Part model, mm, in its own coordinate system. A direction names the side the tool comes from. Coordinates: 2 decimals unless noted, no trailing zeros. Write each loop counter-clockwise with the first axis right and the second up, starting at its lowest first coordinate (ties: lowest second). Pieces come first, ordered by that corner, then holes. Notation, with made-up numbers: (63.25, -14.5) - (86.25, -14.5) arc R3 ccw to (86.25, -10.5) - close; hole circle Ø11 at (76.5, -39.5). An arc over 180 degrees is marked (long way). Write each question's results on one line, items separated by ' | '.
from build123d import *

# Parameters (mm, degrees)
F1_DEPTH = 88.9
F2_W     = 6.731
F2_H     = 6.731
F3_DEPTH = 49.5578889657
F4_ANGLE = 45
F5_ANGLE = 90
F6_ANGLE = 90


with BuildPart() as f1:
    # F0 (on Top) → F1 (new body)
    with BuildSketch(Plane.XY):
        Polygon((-10.7315, -10.7315), (-10.7315, 10.2235), (10.2235, 10.2235), (17.0815, 17.0815), (-0.8790122421, 35.0420122421), (-35.0420122421, 0.8790122421), (-17.0815, -17.0815), align=None)
    extrude(amount=F1_DEPTH)

    # F2 (on face) → F3 (cut, through all)
    with BuildSketch(Plane(origin=(-17.9605122421, 17.9605122421, 0), x_dir=(-0.7071067812, -0.7071067812, 0), z_dir=(-0.7071067812, 0.7071067812, 0))):
        with Locations((0, 44.323)):
            Rectangle(F2_W, F2_H)
    extrude(amount=-F3_DEPTH, mode=Mode.SUBTRACT)


with BuildPart() as f1_1:
    # F4: moved
    add(f1.part.rotate(Axis((-10.7315, 10.2235, 20.47875), (0, 0, -1)), F4_ANGLE))


with BuildPart() as f1_2:
    # F5: moved
    add(f1_1.part.rotate(Axis((-10.3722897552, 20.8060774002, 0), (-1, 0, 0)), F5_ANGLE))


with BuildPart() as f6_1:
    # F6: copy of F1
    add(f1_2.part.rotate(Axis((13.7845992105, 20.8060774002, 12.7), (0, 0, 1)), F6_ANGLE))


with BuildPart() as f6_1_1:
    # F7: moved
    add(f6_1.part.moved(Location((19.05, 0, 0))))


solid = f1_2.part
(1) Saw through at A-A on x = -9. Write the cut outline in (y, z).
Return value:
outline: (20.81, 0) - (61.76, 0) - (61.76, 12.31) - (20.81, 12.31) - close; (68.49, 0) - (109.71, 0) - (109.71, 12.31) - (68.49, 12.31) - close
(2) 3-axis set-ups, long thin cutter, end or side, ignore diameter. For faces 1 (the flat face through (9, 65, 25.4)), 2 (the flat face through (-3.427, 64.634, 17.888)), 3 (the flat face through (-13.738, 65, 7)): which of +Z, -Z, +X, -X, +Y, -Y reach the whole face in a straight line?
Return value:
face 1: +Z, +X, -X, +Y, -Y | face 2: +Z, +Y, -Y | face 3: +Z, -Z
(3) Wall check: line 1 (Y direction, x = -8, z = 1.5); line 2 (X direction, y = 67, z = 11.5); line 3 (X direction, y = 73.5, z = 20). Give the ranges that are in metal, low to high. Write a range as from..to.
Return value:
line 1: y = 20.81..61.76, 68.49..109.71 | line 2: x = -34.53..-13.74, -7.01..13.78 | line 3: x = -34.53..-20.15, -1.31..13.78
(4) Saw through at C-C on y = 39. Write the cut outline in (x, z), then the cut area to 3 significant figures.
Return value:
outline: (-34.53, 0) - (13.78, 0) - (13.78, 25.4) - (4.09, 25.4) - (-10.73, 10.58) - (-25.55, 25.4) - (-34.53, 25.4) - close | area: 1,010 mm^2
(5) Saw through at D-D on x = -21.5. Write the cut outline in (y, z), then the cut area to 3 significant figures.
Return value:
outline: (20.81, 0) - (109.71, 0) - (109.71, 21.35) - (20.81, 21.35) - close | area: 1,900 mm^2
(6) Saw through at B-B on z = 23.5. Write the cut outline in (x, y).
Return value:
outline: (-34.53, 20.81) - (-23.65, 20.81) - (-23.65, 109.71) - (-34.53, 109.71) - close; (2.19, 20.81) - (13.78, 20.81) - (13.78, 109.71) - (2.19, 109.71) - close
(7) Two-plate mould, pull along Y, no slides. Class faces 4 (the flat face through (-18.244, 64.634, 18.095)), 5 (the flat face through (-10, 109.706, 10)), 6 (the flat face through (-10, 61.764, 5)), 7 (the flat face through (-10, 68.495, 5)): released by +Y, released by -Y, zero draft, split by the parting line, or undercut.
Return value:
face 4: zero draft | face 5: released by +Y | face 6: undercut | face 7: undercut
